from build123d import *

# Parameters (mm, degrees)
PAD_DEPTH            = 17
SKETCH001_R          = 31.125
HOLE_DEPTH           = 15.5
SKETCH003_R          = 5.5
POCKET_DEPTH         = 100
POCKET_DEPTH_BACK    = 100
SKETCH010_R          = 5.5
PAD004_DEPTH         = 7.01
SKETCH011_R          = 4
POCKET003_DEPTH      = 100
POCKET003_DEPTH_BACK = 100
CHAMFER001_SIZE      = 2
CHAMFER002_SIZE      = 5
PAD007_DEPTH         = 3.3
POLARPATTERN_COUNT   = 4
FILLET_R             = 1


with BuildPart() as part:
    # Sketch → Pad (new body)
    with BuildSketch(Plane.XY):
        Polygon((-29.250775, 16.887943), (-33.775885, 0), (-29.250775, -16.887943), (-16.887943, -29.250775), (0, -33.775885), (16.887943, -29.250775), (29.250775, -16.887943), (33.775885, 0), (29.250775, 16.887943), (16.887943, 29.250775), (0, 33.775885), (-16.887943, 29.250775), align=None)
    extrude(amount=PAD_DEPTH)

    # Sketch001 (on Face14 of Pad) → Hole (cut)
    with BuildSketch(Plane.XY.offset(17)):
        Circle(SKETCH001_R)
    extrude(amount=-HOLE_DEPTH, mode=Mode.SUBTRACT)

    # Sketch003 → Pocket (cut, two sides)
    with BuildSketch(Plane.XY) as pocket_sk:
        with Locations((0, 15)):
            Circle(SKETCH003_R)
    extrude(amount=-POCKET_DEPTH, mode=Mode.SUBTRACT)
    extrude(pocket_sk.sketch, amount=POCKET_DEPTH_BACK, mode=Mode.SUBTRACT)

    # Sketch010 → Pad004 (join)
    with BuildSketch(Plane.XY):
        with Locations((0, -15)):
            Circle(SKETCH010_R)
    extrude(amount=PAD004_DEPTH)

    # Sketch011 → Pocket003 (cut, two sides)
    with BuildSketch(Plane.XY) as pocket003_sk:
        with Locations((0, -15)):
            Circle(SKETCH011_R)
    extrude(amount=-POCKET003_DEPTH, mode=Mode.SUBTRACT)
    extrude(pocket003_sk.sketch, amount=POCKET003_DEPTH_BACK, mode=Mode.SUBTRACT)

    # Chamfer001
    chamfer001_edges = [part.edges().sort_by_distance(p)[0] for p in [
        (-4, -15, 0),
    ]]
    chamfer(chamfer001_edges, length=CHAMFER001_SIZE)

    # Chamfer002
    chamfer002_edges = [part.edges().sort_by_distance(p)[0] for p in [
        (-5.5, -15, 1.5),
    ]]
    chamfer(chamfer002_edges, length=CHAMFER002_SIZE)

    # Sketch015 (on Face19 of Chamfer002) → Pad007 (join)
    with BuildSketch(Plane(origin=(23.069359, -23.069359, 0), x_dir=(0.707107, 0.707107, 0), z_dir=(0.707107, -0.707107, 0))):
        Polygon((-8, 15.943219), (7.944127, 16.5), (8, 14.9), (-7.944127, 14.343219), align=None)
    pad007 = extrude(amount=-PAD007_DEPTH)

    # PolarPattern: Pad007 ×4 about axis
    polarpattern_axis = Axis((0, 0, 0), (0, 0, 1))
    for i in range(1, POLARPATTERN_COUNT):
        add(pad007.rotate(polarpattern_axis, i * 360 / POLARPATTERN_COUNT))

    # Fillet
    fillet_edges = [part.edges().sort_by_distance(p)[0] for p in [
        (23.069359, 23.069359, 17),
        (8.443971, 31.51333, 17),
        (-8.443971, 31.51333, 17),
        (-23.069359, 23.069359, 17),
        (-31.51333, 8.443971, 17),
        (-31.51333, -8.443971, 17),
        (-23.069359, -23.069359, 17),
        (-8.443971, -31.51333, 17),
        (8.443971, -31.51333, 17),
        (23.069359, -23.069359, 17),
        (31.51333, -8.443971, 17),
        (31.51333, 8.443971, 17),
        (-8.443971, 31.51333, 0),
        (-23.069359, 23.069359, 0),
        (-31.51333, 8.443971, 0),
        (-31.51333, -8.443971, 0),
        (8.443971, 31.51333, 0),
        (23.069359, 23.069359, 0),
        (31.51333, 8.443971, 0),
        (31.51333, -8.443971, 0),
        (23.069359, -23.069359, 0),
        (8.443971, -31.51333, 0),
        (-8.443971, -31.51333, 0),
        (-23.069359, -23.069359, 0),
    ]]
    fillet(fillet_edges, radius=FILLET_R)


solid = part.part
Work out the finished part from the listing and answer in its coordinate system (mm). A direction names the side the tool comes from. Give positions to 0.01 mm unless a question says otherwise; leave off trailing zeros. Order: outer loops, then holes, each group sorted by start corner. A loop starts at its lowest first (then second) coordinate and runs counter-clockwise, first axis right, second up. Notation, with made-up numbers: (-6, 43) -> (3, 43) arc R12 ccw to (3, 62) -> close; hole circle Ø10 at (45.5, -21.75). An arc over 180 degrees is marked (long way). One line per item, written item: value.
Item 1: Find section A-A, the plane z = 5. Give the vertices of the cut face in (x, y) (3 decimals), plus the area to 3 significant figures.
Answer sheet:
outline: (-33.776, 0) -> (-29.251, -16.888) -> (-16.888, -29.251) -> (0, -33.776) -> (16.888, -29.251) -> (29.251, -16.888) -> (33.776, 0) -> (29.251, 16.888) -> (16.888, 29.251) -> (0, 33.776) -> (-16.888, 29.251) -> (-29.251, 16.888) -> close; circle Ø14 at (0, -15); hole circle Ø62.25 at (0, 0); hole circle Ø8 at (0, -15)
area: 483 mm²
Item 2: Flat-ended cylindrical pins translate along their axes: P1, Ø5.5, axis at x = 0.5, y = -12.5, coming from the +Z side; P2, Ø3, axis at y = -2, z = 5, coming from the -X side; P3, Ø10, axis at y = 21, z = 9.5, coming from the -X side; P4, Ø6.5, axis at x = 0, y = -15, coming from the -Z side. Find the tip coordinate at first contact, or state that the pin passes through.
Answer sheet:
P1: z = 7.01
P2: x = -33.64
P3: x = -29.49
P4: through
Item 3: Straight lines are drawn through the part: probe 1 along X at (y, z) = (-15, 5); probe 2 along X at (y, z) = (-15, 4.1); probe 3 along Z at (x, y) = (-11.5, -11.5). For each, find the intervals that lie inside material, in ascending order.
Answer sheet:
probe 1: -29.76 to -27.27, -7 to -4, 4 to 7, 27.27 to 29.76
probe 2: -29.76 to -27.27, -7.9 to -4, 4 to 7.9, 27.27 to 29.76
probe 3: 0 to 1.5
Item 4: Determine the mould class of faces 3 (the flat face through (23.16, -22.98, 8.6)), 4 (the flat face through (-22.98, -23.16, 8.6)), 5 (the flat face through (-4, -17, 7.01)) for opening direction X: released by +X, released by -X, zero draft, split by the parting line, or undercut.
Answer sheet:
face 3: released by +X
face 4: released by -X
face 5: undercut
Item 5: Find section B-B, the plane z = 11.25. Give the vertices of the cut face in (x, y) (3 decimals), plus the area to 3 significant figures.
Answer sheet:
outline: (-33.776, 0) -> (-29.251, -16.888) -> (-16.888, -29.251) -> (0, -33.776) -> (16.888, -29.251) -> (29.251, -16.888) -> (33.776, 0) -> (29.251, 16.888) -> (16.888, 29.251) -> (0, 33.776) -> (-16.888, 29.251) -> (-29.251, 16.888) -> close; hole circle Ø62.25 at (0, 0)
area: 379 mm²
Item 6: A tool of negligible diameter and unlimited length cuts with its end or side. For faces 1 (the cylindrical face through (-1.19, -20.37, 6.75)), 2 (the flat face through (-8.562, -31.482, 8.395)), from which of +Z, -Z, +X, -X, +Y, -Y can it reach the whole face along a straight path? Write none if from no direction.
Answer sheet:
face 1: +Z
face 2: +Z, -Z, -X, -Y
